Model file for the job. Use its own axes, mm. A direction names the side the tool comes from. Round coordinates to 2 decimals unless told otherwise and drop trailing zeros. Order: outer loops, then holes, each group sorted by start corner. A loop starts at its lowest first (then second) coordinate and runs counter-clockwise, first axis right, second up. Notation, with made-up numbers: M -33.5,-9.5 L 7.5,-9.5 A14 cw 7.5,12.5 Z; hole C 42,40 d7. An arc over 180 degrees is marked long. Return JSON: item names as keys, results as strings. Group by question number.
Item 1: Slice it at C-C on y = 3.8. Write the cut outline in (x, z).
Item 2: Which spindle directions (+Z, -Z, +X, -X, +Y, -Y) get a long thin tool onto all of the face, cutting with end or side? Do faces 4 (the face through (18, 2, 0)), 5 (the face through (-3.1, 1, -8.2)), 6 (the face through (-18, 2, 0)), 7 (the face through (0, 2, 0)). Say none if no direction does.
Item 3: Slice it at A-A on x = 8.5. Write the cut outline in (y, z), then the cut area to 3 significant figures.
Item 4: Slice it at B-B on z = 0. Write the cut outline in (x, y).
Item 5: Pin check, flat tips, straight feed: pin 1 Ø1.5 at (x, z) = (-10.5, 1.5) entering from +Y; pin 2 Ø10 at (x, z) = (0.5, 0.5) entering from -Y; pin 3 Ø1.6 at (x, y) = (1.5, 2.5) entering from +Z. Stop position of each tip, or through.
Item 6: Probe line 1 along X through (y, z) = (0.3, -8); line 2 along Z through (x, y) = (6, 0.3); line 3 along X through (y, z) = (0.5, -7.25). List the from-to ranges inside material, lowest first.
Item 7: Pull direction X, two halves, no side cores. Call faces 1 (the face through (0, 5.8, 0)), 2 (the face through (-17, 1, 0)), 3 (the face through (-20, 0.5, 0.1)): pulls with the +X half, pulls with the -X half, needs draft (parallel to the pull), parting line crosses it, or undercut.
Item 8: Slice it at D-D on x = -12. Write the cut outline in (y, z).
from build123d import *

# Parameters (mm, degrees)
SKETCH_1_W          = 40
SKETCH_1_H          = 20
EXTRUDE_1_DEPTH     = 1
SKETCH_2_R          = 1
CUT_EXTRUDE_1_DEPTH = 1
EXTRUDE_2_DEPTH     = 2
SHELL_2_DEPTH       = 2
SKETCH_4_R          = 7.25
EXTRUDE_3_DEPTH     = 2.8


# Read off the part's stored shape, not the designer's step: 抽壳2
with BuildPart() as part:
    # 草图1 → 凸台-拉伸1 (new body)
    with BuildSketch(Plane(origin=(0, 0, 0), x_dir=(1, 0, 0), z_dir=(0, 1, 0))):
        Rectangle(SKETCH_1_W, SKETCH_1_H)
    extrude(amount=EXTRUDE_1_DEPTH)

    # 草图2 → 切除-拉伸1 (cut)
    with BuildSketch(Plane(origin=(0, 1, 0), x_dir=(1, 0, 0), z_dir=(0, 1, 0))):
        with Locations(Location((-18, 8, 0), (0, 0, 270))):
            Circle(SKETCH_2_R)
        with Locations(Location((18, 8, 0), (0, 0, 90))):
            Circle(SKETCH_2_R)
        with Locations(Location((18, -8, 0), (0, 0, 270))):
            Circle(SKETCH_2_R)
        with Locations(Location((-18, -8, 0), (0, 0, 90))):
            Circle(SKETCH_2_R)
    extrude(amount=-CUT_EXTRUDE_1_DEPTH, mode=Mode.SUBTRACT)

    # 草图3 → 凸台-拉伸2 (add)
    with BuildSketch(Plane(origin=(0, 1, 0), x_dir=(1, 0, 0), z_dir=(0, 1, 0))):
        with BuildLine():
            Line((-10, 8), (10, 8))
            ThreePointArc((10, 8), (18, 0), (10, -8))
            Line((10, -8), (-10, -8))
            ThreePointArc((-10, -8), (-18, 0), (-10, 8))
        make_face()
    extrude(amount=EXTRUDE_2_DEPTH)

    # 抽壳2 outline → 抽壳2 (cut)
    with BuildSketch(Plane(origin=(0, 0, 0), x_dir=(1, 0, 0), z_dir=(0, 1, 0))):
        with BuildLine():
            ThreePointArc((-10, 7), (-17, 0), (-10, -7))
            Line((-10, -7), (10, -7))
            ThreePointArc((10, -7), (17, 0), (10, 7))
            Line((10, 7), (-10, 7))
        make_face()
    extrude(amount=SHELL_2_DEPTH, mode=Mode.SUBTRACT)

    # 草图4 → 凸台-拉伸3 (add)
    with BuildSketch(Plane(origin=(0, 3, 0), x_dir=(1, 0, 0), z_dir=(0, 1, 0))):
        with Locations(Location((0, 0, 0), (0, 0, 270))):
            Circle(SKETCH_4_R)
    extrude(amount=EXTRUDE_3_DEPTH)


solid = part.part
Output values:
{
 "1": {"outline": "C 0,0 d14.5"},
 "2": {"face 4": "+X, +Y", "face 5": "+Y", "face 6": "-X, +Y", "face 7": "-Y"},
 "3": {"outline": "M 0,-10 L 1,-10 L 1,-8 L 3,-8 L 3,8 L 1,8 L 1,10 L 0,10 L 0,7 L 2,7 L 2,-7 L 0,-7 Z", "area": "24.0 mm²"},
 "4": {"outline": "M -20,0 L -17,0 L -17,2 L 17,2 L 17,0 L 20,0 L 20,1 L 18,1 L 18,3 L 7.25,3 L 7.25,5.8 L -7.25,5.8 L -7.25,3 L -18,3 L -18,1 L -20,1 Z"},
 "5": {"pin 1": "y = 3", "pin 2": "y = 2", "pin 3": "z = 8"},
 "6": {"line 1": "-20 to -19, -17 to 17, 19 to 20", "line 2": "-10 to -7, 7 to 10", "line 3": "-20 to -18.66, -17.34 to 17.34, 18.66 to 20"},
 "7": {"face 1": "needs draft", "face 2": "undercut", "face 3": "pulls with the -X half"},
 "8": {"outline": "M 0,-10 L 1,-10 L 1,-7.75 L 3,-7.75 L 3,7.75 L 1,7.75 L 1,10 L 0,10 L 0,6.71 L 2,6.71 L 2,-6.71 L 0,-6.71 Z"}
}
